from build123d import *

# Parameters (mm, degrees)
F0_W     = 30
F0_H     = 6
F1_DEPTH = 150
F2_R     = 0.8
F2_R_2   = 4
F3_DEPTH = 6
F4_W     = 3
F4_H     = 50
F5_DEPTH = 30
F6_W     = 4.599998
F6_H     = 4.599998
F6_W_2   = 4.6
F6_H_2   = 4.6
F7_DEPTH = 3
F8_R     = 10.5
F9_DEPTH = 3


with BuildPart() as f1:
    # F0 (on Top) → F1 (new body)
    with BuildSketch(Plane.XY):
        Rectangle(F0_W, F0_H)
    extrude(amount=F1_DEPTH)

    # F2 (on face) → F3 (cut, through all)
    with BuildSketch(Plane.XZ.offset(3)):
        with Locations((0, 146.2)):
            Circle(F2_R)
        with Locations((0, 138.2)):
            Circle(F2_R_2)
        with Locations((-5.656854, 143.856854)):
            Circle(F2_R)
        with Locations((-8, 138.2)):
            Circle(F2_R)
        with Locations((-5.656854, 132.543146)):
            Circle(F2_R)
        with Locations((0, 130.2)):
            Circle(F2_R)
        with Locations((5.656854, 132.543146)):
            Circle(F2_R)
        with Locations((8, 138.2)):
            Circle(F2_R)
        with Locations((5.656854, 143.856854)):
            Circle(F2_R)
    extrude(amount=-F3_DEPTH, mode=Mode.SUBTRACT)

    # F4 (on face) → F5 (cut, through all)
    with BuildSketch(Plane(origin=(-15, 0, 0), x_dir=(0, -1, 0), z_dir=(-1, 0, 0))):
        with Locations((1.5, 25)):
            Rectangle(F4_W, F4_H)
    extrude(amount=-F5_DEPTH, mode=Mode.SUBTRACT)

    # F6 (on face) → F7 (join)
    with BuildSketch(Plane.XZ):
        with Locations((7.5, 37.5)):
            Rectangle(F6_W, F6_H)
        with Locations((-7.5, 37.5)):
            Rectangle(F6_W, F6_H)
        with Locations((-7.5, 7.5)):
            Rectangle(F6_W_2, F6_H_2)
        with Locations((7.5, 7.5)):
            Rectangle(F6_W_2, F6_H_2)
    extrude(amount=F7_DEPTH)

    # F8 (on face) → F9 (cut)
    with BuildSketch(Plane.XZ.offset(3)):
        with Locations((0, 138.2)):
            Circle(F8_R)
    extrude(amount=-F9_DEPTH, mode=Mode.SUBTRACT)


solid = f1.part
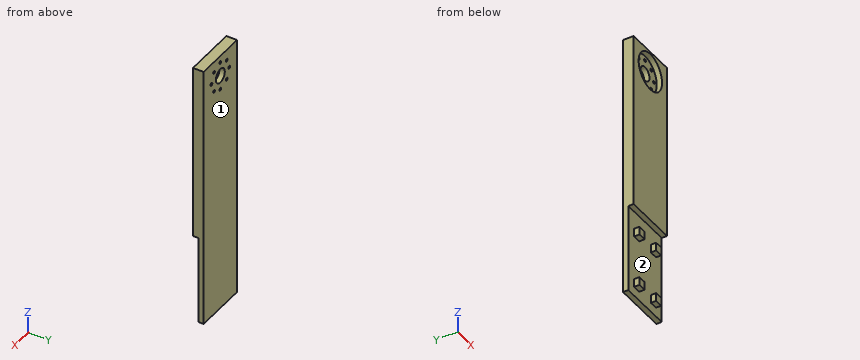
Geometry check sheet. Reference: the model listing, model coordinates, mm. Face numbers are marked on the shaded views. Round coordinates to 2 decimals unless told otherwise and drop trailing zeros. Loops run counter-clockwise (first coordinate to the right, second up) from the corner with the lowest first, then second, coordinate; pieces in that order, holes last. Notation, with made-up numbers: (-35.5, 77.25) -> (11.5, 77.25) arc R16 cw to (11.5, 104.25) -> close; hole circle Ø2 at (62, 75.25). An arc over 180 degrees is marked (long way). Answer as a JSON object with one key per item and string values. Group by question number.
Item 1: Release check for a two-part mould opening along Z. For the marked faces 1 and 2 record: pulls with the +Z half, pulls with the -Z half, needs draft (parallel to the pull), parting line crosses it, or undercut.
Item 2: Thickness scan on line 1 along Z through (x, y) = (5.75, 1.2); line 2 along Z through (x, y) = (0, 0.85); line 3 along Z through (x, y) = (-6.25, 1.2). Record the ranges inside material, lowest first.
Item 3: Depth check by flat-ended pin: pin 1 Ø0.9 at (x, y) = (7, -1) entering from -Z; pin 2 Ø1.5 at (y, z) = (-2, 7.5) entering from +X; pin 3 Ø2.5 at (y, z) = (-1, 37) entering from +X; pin 4 Ø1.3 at (x, z) = (5.66, 132.54) entering from -Y. Enter the tip coordinate at first touch or a pass-through.
Item 4: Cross-section at C-C, the plane z = 18.5. Record the cut outline in (x, y).
Item 5: Cross-section at A-A, the plane y = -1.05. Record the cut outline in (x, z), plus the area to 3 significant figures.
Item 6: Cross-section at B-B, the plane x = -11.75. Record the cut outline in (y, z).
Determined:
{
 "1": {"face 1": "needs draft", "face 2": "undercut"},
 "2": {"line 1": "z = 0 to 131.75, 133.34 to 143.06, 144.65 to 150", "line 2": "z = 0 to 129.4, 131 to 134.2, 142.2 to 145.4, 147 to 150", "line 3": "z = 0 to 132.01, 133.08 to 143.32, 144.39 to 150"},
 "3": {"pin 1": "stops at z = 5.2", "pin 2": "stops at x = 9.8", "pin 3": "stops at x = 15", "pin 4": "passes through"},
 "4": {"outline": "(-15, 0) -> (15, 0) -> (15, 3) -> (-15, 3) -> close"},
 "5": {"outline": "(-15, 50) -> (15, 50) -> (15, 150) -> (-15, 150) -> close; (-9.8, 5.2) -> (-5.2, 5.2) -> (-5.2, 9.8) -> (-9.8, 9.8) -> close; (-9.8, 35.2) -> (-5.2, 35.2) -> (-5.2, 39.8) -> (-9.8, 39.8) -> close; (5.2, 5.2) -> (9.8, 5.2) -> (9.8, 9.8) -> (5.2, 9.8) -> close; (5.2, 35.2) -> (9.8, 35.2) -> (9.8, 39.8) -> (5.2, 39.8) -> close; hole circle Ø21 at (0, 138.2)", "area": "2,740 mm²"},
 "6": {"outline": "(-3, 50) -> (0, 50) -> (0, 0) -> (3, 0) -> (3, 150) -> (-3, 150) -> close"}
}
